Could you check a few things on this model? Use its own coordinates, in mm. A direction names the side the tool comes from. Give positions to 0.01 mm unless a question says otherwise; leave off trailing zeros. Order: outer loops, then holes, each group sorted by start corner. A loop starts at its lowest first (then second) coordinate and runs counter-clockwise, first axis right, second up. Notation, with made-up numbers: M -7,31.5 L 30,31.5 A28 cw 30,65.5 Z; hole C 9,22.25 d10. An arc over 180 degrees is marked long. Return JSON: item names as keys, results as strings. Group by question number.
```python
from build123d import *

# Parameters (mm, degrees)
F1_DEPTH = 20
F2_W     = 48
F2_H     = 2
F3_DEPTH = 3.5
F5_DEPTH = 2


with BuildPart() as f1:
    # F0 (on Front) → F1 (new body)
    with BuildSketch(Plane.XZ):
        Polygon((26, -7.568409), (26, 12.431591), (-26, 12.431591), (-26, -7.568409), (-24.5, -7.568409), (-22.5, -4.568409), (-24, -4.568409), (-24, 10.431591), (24, 10.431591), (24, -4.568409), (22.5, -4.568409), (24.5, -7.568409), align=None)
    extrude(amount=F1_DEPTH)

    # F2 (on face) → F3 (join)
    with BuildSketch(Plane(origin=(0, 0, 10.431591), x_dir=(1, 0, 0), z_dir=(0, 0, -1))):
        with Locations((0, 1)):
            Rectangle(F2_W, F2_H)
        with Locations((0, 11)):
            Rectangle(F2_W, F2_H)
    extrude(amount=F3_DEPTH)

    # F4 (on face) → F5 (join)
    with BuildSketch(Plane.XZ.offset(20)):
        with BuildLine():
            Line((26, 12.431591), (-26, 12.431591))
            Line((-26, 12.431591), (-26, 4.431591))
            Line((-26, 4.431591), (-20, 4.431591))
            ThreePointArc((-20, 4.431591), (-17.5, 6.931591), (-15, 4.431591))
            Line((-15, 4.431591), (-12.109772, 4.431591))
            ThreePointArc((-12.109772, 4.431591), (-7.5, 6.931591), (-2.890228, 4.431591))
            Line((-2.890228, 4.431591), (2.890228, 4.431591))
            ThreePointArc((2.890228, 4.431591), (7.5, 6.931591), (12.109772, 4.431591))
            Line((12.109772, 4.431591), (15, 4.431591))
            ThreePointArc((15, 4.431591), (17.5, 6.931591), (20, 4.431591))
            Line((20, 4.431591), (26, 4.431591))
            Line((26, 4.431591), (26, 12.431591))
        make_face()
    extrude(amount=-F5_DEPTH)


solid = f1.part
```
1. If we mould it in two halves opening along Y, with no side actions, what happens to faces 1 (the flat face through (0, -1, 6.932)), 2 (the flat face through (0, -2, 9)), 3 (the flat face through (0, 0, 8))? For each: pulls with the +Y half, pulls with the -Y half, needs draft (parallel to the pull), parting line crosses it, or undercut.
2. For pin 1 (5 mm diameter, centred on x = -17.5, z = 6.5, fed in from +Y); pin 2 (4 mm diameter, centred on x = 8, y = -6, fed in from -Z); pin 3 (1.6 mm diameter, centred on x = -22.5, y = -19, fed in from -Z); pin 4 (0.6 mm diameter, centred on x = 0.5, y = -19, fed in from -Z), each with a flat end and sliding along its axis, tell me the tip position at first contact or that it passes through.
3. Imagine slicing it at A-A, the plane z = -2. Please give me the cut outline in (x, y), plus the area to 3 significant figures.
4. Imagine slicing it at D-D, the plane z = 6.25. Please give me the cut outline in (x, y), plus the area to 3 significant figures.
5. Imagine slicing it at B-B, the plane y = -6. Please give me the cut outline in (x, z), plus the area to 3 significant figures.
6. Which directions (+Z, -Z, +X, -X, +Y, -Y) give clear straight access to the entire face, cutting with the end or side of a thin tool? Please do faces 4 (the flat face through (-24, -10, 3)), 5 (the flat face through (25, -10, -7.568)), 6 (the flat face through (-26, -10, 3)), 7 (the flat face through (-23.514, -9.86, -6.089)), 8 (the flat face through (22, -19, 4.432)).
7. Imagine slicing it at C-C, the plane x = -2. Please give me the cut outline in (y, z).
8. I need wall thicknesses on L1, parallel to Y at x = 2.5, z = 10; L2, parallel to X at y = -16, z = -2; L3, parallel to Z at x = -0.5, y = -16.75. Which ranges of each line are inside material? Lowest first, please. Write a range as from..to.
Values:
{
 "1": {"face 1": "needs draft", "face 2": "undercut", "face 3": "pulls with the +Y half"},
 "2": {"pin 1": "stops at y = 0", "pin 2": "stops at z = 10.43", "pin 3": "stops at z = -5.77", "pin 4": "stops at z = 4.43"},
 "3": {"outline": "M -26,-20 L -24,-20 L -24,0 L -26,0 Z; M 24,-20 L 26,-20 L 26,0 L 24,0 Z", "area": "80.0 mm²"},
 "4": {"outline": "M -26,-20 L -19.22,-20 L -19.22,-18 L -24,-18 L -24,0 L -26,0 Z; M -15.78,-20 L -10.15,-20 L -10.15,-18 L -15.78,-18 Z; M -4.85,-20 L 4.85,-20 L 4.85,-18 L -4.85,-18 Z; M 10.15,-20 L 15.78,-20 L 15.78,-18 L 10.15,-18 Z; M 19.22,-20 L 26,-20 L 26,0 L 24,0 L 24,-18 L 19.22,-18 Z", "area": "141 mm²"},
 "5": {"outline": "M -26,-7.57 L -24.5,-7.57 L -22.5,-4.57 L -24,-4.57 L -24,10.43 L 24,10.43 L 24,-4.57 L 22.5,-4.57 L 24.5,-7.57 L 26,-7.57 L 26,12.43 L -26,12.43 Z", "area": "179 mm²"},
 "6": {"face 4": "none", "face 5": "-Z, +X, -X, +Y, -Y", "face 6": "+Z, -Z, -X, +Y, -Y", "face 7": "-Z, +Y, -Y", "face 8": "+Y, -Y"},
 "7": {"outline": "M -20,4.43 L -18,4.43 L -18,10.43 L -12,10.43 L -12,6.93 L -10,6.93 L -10,10.43 L -2,10.43 L -2,6.93 L 0,6.93 L 0,12.43 L -20,12.43 Z"},
 "8": {"L1": "y = -20..-18, -12..-10, -2..0", "L2": "x = -26..-24, 24..26", "L3": "z = 10.43..12.43"}
}
